```python
from build123d import *

# Parameters (mm, degrees)
SALIENTE_EXTRUIR1_DEPTH = 7.5
SALIENTE_EXTRUIR2_DEPTH = 15
CROQUIS7_R              = 3.5
CORTAR_EXTRUIR4_DEPTH   = 13.8
CORTAR_EXTRUIR5_START   = -3
CORTAR_EXTRUIR5_DEPTH   = 10
CHAFL_N4_SIZE           = 4
CHAFL_N5_SIZE           = 0.8


with BuildPart() as part:
    # Croquis1 → Saliente-Extruir1 (new body, symmetric)
    with BuildSketch(Plane.XY):
        with BuildLine():
            Line((-8.9, 4), (-4.920420362, 7.979579638))
            ThreePointArc((-4.920420362, 7.979579638), (-3.998499164, 5.705173276), (-2.1, 4.15))
            Line((-2.1, 4.15), (0, 4.15))
            Line((0, 4.15), (0, -4.15))
            ThreePointArc((0, -4.15), (-4.800362316, -3.215771009), (-8.9, -0.549456506))
            Line((-8.9, -0.549456506), (-8.9, 4))
        make_face()
    extrude(amount=SALIENTE_EXTRUIR1_DEPTH, both=True)

    # Croquis6 → Saliente-Extruir2 (add, through all)
    with BuildSketch(Plane(origin=(0, 0, -7.5), x_dir=(-1, 0, 0), z_dir=(0, 0, -1))):
        Polygon((0, -4.15), (0, -7.15), (-3, -7.15), (-6, -4.15), (-22.5, -4.15), (-22.5, 5.65), (-1.5, 5.65), (0, 4.15), align=None)
    extrude(amount=-SALIENTE_EXTRUIR2_DEPTH)

    # Croquis7 → Cortar-Extruir4 (cut, through all)
    with BuildSketch(Plane(origin=(0, 5.65, 0), x_dir=(1, 0, 0), z_dir=(0, 1, 0))):
        with Locations((15, 0)):
            Circle(CROQUIS7_R)
    extrude(amount=-CORTAR_EXTRUIR4_DEPTH, mode=Mode.SUBTRACT)

    # Croquis8 → Cortar-Extruir5 (cut)
    with BuildSketch(Plane(origin=(0, 5.65, 0), x_dir=(1, 0, 0), z_dir=(0, 1, 0)).offset(CORTAR_EXTRUIR5_START)):
        Polygon((15, 5.658032638), (10.1, 2.829016319), (10.1, -2.829016319), (15, -5.658032638), (19.9, -2.829016319), (19.9, 2.829016319), align=None)
    extrude(amount=-CORTAR_EXTRUIR5_DEPTH, mode=Mode.SUBTRACT)

    # Chaflán4
    chafl_n4_edges = [part.edges().sort_by_distance(p)[0] for p in [
        (22.5, 0.75, 7.5),
        (22.5, 0.75, -7.5),
    ]]
    chamfer(chafl_n4_edges, length=CHAFL_N4_SIZE)

    # Chaflán5
    chafl_n5_edges = [part.edges().sort_by_distance(p)[0] for p in [
        (11.5, 5.65, 0),
        (12.55, -4.15, -4.243524479),
        (10.1, -4.15, 0),
        (12.55, -4.15, 4.243524479),
        (17.45, -4.15, 4.243524479),
        (19.9, -4.15, 0),
        (17.45, -4.15, -4.243524479),
    ]]
    chamfer(chafl_n5_edges, length=CHAFL_N5_SIZE)


solid = part.part
```
Build history of the part. All positions in model axes, mm. A direction names the side the tool comes from. Give positions to 0.01 mm unless a question says otherwise; leave off trailing zeros. Loops run counter-clockwise (first coordinate to the right, second up) from the corner with the lowest first, then second, coordinate; pieces in that order, holes last.
1) Band-saw the part on D-D on y = -5.5. List the corners of the cut face in (x, z).
Values follow:
outline: (0, -7.5) - (4.65, -7.5) - (4.65, 7.5) - (0, 7.5) - close
2) Probe line 1 along Z through (x, y) = (15, 3.75); line 2 along Y through (x, z) = (12.5, 6); line 3 along X through (y, z) = (3.4, 0). List the from-to ranges inside material, lowest first.
Values follow:
line 1: z = -7.5 to -3.5, 3.5 to 7.5
line 2: y = -4.15 to 5.65
line 3: x = -8.9 to 11.5, 18.5 to 22.5
3) Band-saw the part on C-C on z = -5. List the corners of the cut face in (x, y).
Values follow:
outline: (-8.9, -0.55) arc R12.8 ccw to (0, -4.15) - (0, -7.15) - (3, -7.15) - (6, -4.15) - (12.26, -4.15) - (13.86, -3.35) - (13.86, 2.65) - (16.14, 2.65) - (16.14, -3.35) - (17.74, -4.15) - (21, -4.15) - (21, 5.65) - (1.5, 5.65) - (0, 4.15) - (-2.1, 4.15) arc R4.97 cw to (-4.92, 7.98) - (-8.9, 4) - close
4) 3-axis set-ups, long thin cutter, end or side, ignore diameter. For faces 1 (the face through (-4.019, 5.733, 0.105)), 2 (the face through (0, -6, 0)), 3 (the face through (10, 5.65, 0)), 4 (the face through (12.58, -0.31, -4.26)): which of +Z, -Z, +X, -X, +Y, -Y reach the whole face in a straight line?
Values follow:
face 1: +Z, -Z, +Y
face 2: +Z, -Z, -X, -Y
face 3: +Z, -Z, +X, +Y
face 4: -Y
5) Band-saw the part on A-A on z = 0. List the corners of the cut face in (x, y), then the cut area to 3 significant figures.
Values follow:
outline: (-8.9, -0.55) arc R12.8 ccw to (0, -4.15) - (0, -7.15) - (3, -7.15) - (6, -4.15) - (9.3, -4.15) - (10.1, -3.35) - (10.1, 2.65) - (11.5, 2.65) - (11.5, 4.85) - (10.7, 5.65) - (1.5, 5.65) - (0, 4.15) - (-2.1, 4.15) arc R4.97 cw to (-4.92, 7.98) - (-8.9, 4) - close; (18.5, 2.65) - (19.9, 2.65) - (19.9, -3.35) - (20.7, -4.15) - (22.5, -4.15) - (22.5, 5.65) - (19.3, 5.65) - (18.5, 4.85) - close
area: 219 mm2
6) Band-saw the part on B-B on y = 0. List the corners of the cut face in (x, z).
Values follow:
outline: (-8.9, -7.5) - (18.5, -7.5) - (22.5, -3.5) - (22.5, 3.5) - (18.5, 7.5) - (-8.9, 7.5) - close; hole (10.1, -2.83) - (15, -5.66) - (19.9, -2.83) - (19.9, 2.83) - (15, 5.66) - (10.1, 2.83) - close
7) Two-plate mould, pull along Z, no slides. Class faces 5 (the face through (21, 1, -5)), 6 (the face through (-4.74, -3.24, 0.11)), 7 (the face through (20.29, -3.74, 0.05)): released by +Z, released by -Z, zero draft, split by the parting line, or undercut.
Values follow:
face 5: released by -Z
face 6: zero draft
face 7: undercut
8) Drop flat-ended pins along their axis: P1, Ø0.9, axis at y = -6.5, z = -1.5, coming from the -X side; P2, Ø6.5, axis at x = 15, z = 0, coming from the +Y side (3 decimals); P3, Ø1.1, axis at x = -1.5, z = 1.5, coming from the +Y side; P4, Ø2, axis at x = 7.5, z = 2.5, coming from the -Y side. Give the stop position or say it passes through.
Values follow:
P1: stops at x = 0
P2: passes through
P3: stops at y = 4.15
P4: stops at y = -4.15
